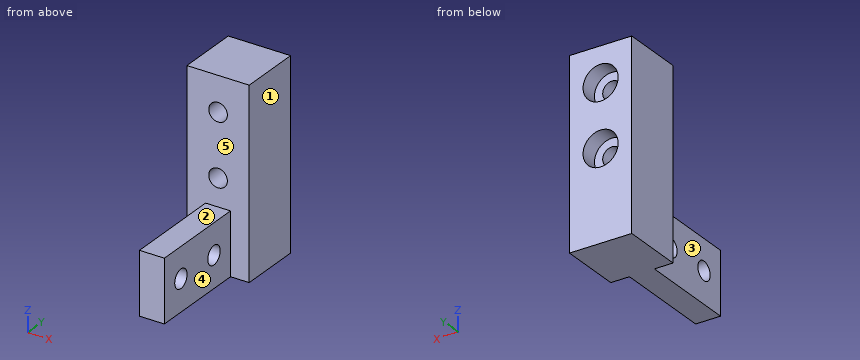
from build123d import *

# Parameters (mm, degrees)
SKETCH1_W                                      = 38.1
SKETCH1_H                                      = 12.7
BOSS_EXTRUDE1_DEPTH                            = 12.7
SKETCH2_W                                      = 12.7
SKETCH2_H                                      = 12.7
BOSS_EXTRUDE2_DEPTH                            = 20.32
SKETCH3_W                                      = 3.81
SKETCH3_H                                      = 20.32
CUT_EXTRUDE1_DEPTH                             = 12.7
F_6_CLEARANCE_HOLE1_D                          = 3.7973
F_6_CLEARANCE_HOLE1_DEPTH                      = 10.16
F_6_CLEARANCE_HOLE1_TIP                        = 1.140824014
CBORE_FOR_6_SOCKET_HEAD_CAP_SCREW1_D           = 3.7973
CBORE_FOR_6_SOCKET_HEAD_CAP_SCREW1_CBORE_D     = 7.14502
CBORE_FOR_6_SOCKET_HEAD_CAP_SCREW1_CBORE_DEPTH = 3.5052


with BuildPart() as part:
    # Sketch1 → Boss-Extrude1 (new body)
    with BuildSketch(Plane(origin=(0, 0, 0), x_dir=(0, 0, -1), z_dir=(1, 0, 0))):
        with Locations((19.05, -6.35)):
            Rectangle(SKETCH1_W, SKETCH1_H)
    extrude(amount=BOSS_EXTRUDE1_DEPTH)

    # Sketch2 → Boss-Extrude2 (add)
    with BuildSketch(Plane.XZ.offset(12.7)):
        with Locations((6.35, -31.75)):
            Rectangle(SKETCH2_W, SKETCH2_H)
    extrude(amount=BOSS_EXTRUDE2_DEPTH)

    # Sketch3 → Cut-Extrude1 (cut)
    with BuildSketch(Plane(origin=(0, 0, -38.1), x_dir=(-1, 0, 0), z_dir=(0, 0, -1))):
        with Locations((-10.795, -22.86)):
            Rectangle(SKETCH3_W, SKETCH3_H)
        with Locations((-1.905, -22.86)):
            Rectangle(SKETCH3_W, SKETCH3_H)
    extrude(amount=-CUT_EXTRUDE1_DEPTH, mode=Mode.SUBTRACT)

    # #6 Clearance Hole1
    with Locations(Plane(origin=(8.89, 0, 0), x_dir=(0, 0, -1), z_dir=(1, 0, 0))):
        with Locations((31.647977642, -17.78), (31.647977642, -27.94), (44.509550176, -23.706107059)):
            Hole(F_6_CLEARANCE_HOLE1_D / 2, depth=F_6_CLEARANCE_HOLE1_DEPTH)
            with Locations((0, 0, -(F_6_CLEARANCE_HOLE1_DEPTH + F_6_CLEARANCE_HOLE1_TIP / 2))):  # 118° drill point
                Cone(0, F_6_CLEARANCE_HOLE1_D / 2, F_6_CLEARANCE_HOLE1_TIP, mode=Mode.SUBTRACT)

    # CBORE for #6 Socket Head Cap Screw1 (through all)
    with Locations(Plane(origin=(0, 0, 0), x_dir=(1, 0, 0), z_dir=(0, 1, 0))):
        with Locations((6.35, 7.112), (6.35, 19.812)):
            CounterBoreHole(CBORE_FOR_6_SOCKET_HEAD_CAP_SCREW1_D / 2, CBORE_FOR_6_SOCKET_HEAD_CAP_SCREW1_CBORE_D / 2, CBORE_FOR_6_SOCKET_HEAD_CAP_SCREW1_CBORE_DEPTH)


solid = part.part
Verification items for the finished model (mm, model axes). Face numbers are marked on the shaded views. A direction names the side the tool comes from. Round coordinates to 2 decimals unless told otherwise and drop trailing zeros. Order: outer loops, then holes, each group sorted by start corner. A loop starts at its lowest first (then second) coordinate and runs counter-clockwise, first axis right, second up.
1. Section check D-D on x = 10.5. Record the cut outline in (y, z), then the cut area to 3 significant figures.
Final values:
outline: (-12.7, -38.1) - (0, -38.1) - (0, 0) - (-12.7, 0) - close
area: 484 mm2
2. Thickness scan on L1, parallel to Z at x = 6.35, y = -9; L2, parallel to Z at x = 8.5, y = -3; L3, parallel to Y at x = 8.5, z = -2.5. Record the ranges inside material, lowest first.
Final values:
L1: z = -38.1 to -21.71, -17.91 to -9.01, -5.21 to 0
L2: z = -38.1 to -22.67, -16.96 to -9.97, -4.26 to 0
L3: y = -12.7 to 0
3. Access from +Z, -Z, +X, -X, +Y, -Y to the whole of each face (thin tool, end or side, straight path). Record for the marked faces 1, 2, 3, 4 and 5.
Final values:
face 1: +Z, -Z, +X, +Y, -Y
face 2: +Z, +X, -X, -Y
face 3: +Z, -Z, -X, -Y
face 4: +Z, -Z, +X, -Y
face 5: +Z, -Y
4. Section check A-A on y = -17.78. Record the cut outline in (x, z), then the cut area to 3 significant figures.
Final values:
outline: (3.81, -38.1) - (8.89, -38.1) - (8.89, -33.55) - (3.81, -33.55) - close; (3.81, -29.75) - (8.89, -29.75) - (8.89, -25.4) - (3.81, -25.4) - close
area: 45.2 mm2
5. Section check C-C on y = -9. Record the cut outline in (x, z), then the cut area to 3 significant figures.
Final values:
outline: (0, -38.1) - (12.7, -38.1) - (12.7, 0) - (0, 0) - close; hole circle Ø3.8 at (6.35, -19.81); hole circle Ø3.8 at (6.35, -7.11)
area: 461 mm2
6. Section check B-B on x = 6.35. Record the cut outline in (y, z), then the cut area to 3 significant figures.
Final values:
outline: (-33.02, -38.1) - (0, -38.1) - (0, -23.38) - (-3.51, -23.38) - (-3.51, -21.71) - (-12.7, -21.71) - (-12.7, -25.4) - (-33.02, -25.4) - close; (-12.7, -17.91) - (-3.51, -17.91) - (-3.51, -16.24) - (0, -16.24) - (0, -10.68) - (-3.51, -10.68) - (-3.51, -9.01) - (-12.7, -9.01) - close; (-12.7, -5.21) - (-3.51, -5.21) - (-3.51, -3.54) - (0, -3.54) - (0, 0) - (-12.7, 0) - close; hole circle Ø3.8 at (-27.94, -31.65); hole circle Ø3.8 at (-17.78, -31.65)
area: 599 mm2
7. Go/stop test with flat-tipped pins: P1, Ø6.5, axis at x = 6.35, z = -7.112, coming from the +Y side; P2, Ø6, axis at x = 6.35, z = -7.112, coming from the -Y side; P3, Ø10, axis at y = -23.5, z = -34.5, coming from the -X side; P4, Ø8, axis at y = -27.5, z = -19, coming from the +X side. Record where each tip stops, or that it passes through.
Final values:
P1: stops at y = -3.51
P2: stops at y = -12.7
P3: stops at x = 3.81
P4: passes through
